```python
from build123d import *

# Parameters (mm, degrees)
SKETCH1_R           = 34.925
BOSS_EXTRUDE1_DEPTH = 3.175
CUT_EXTRUDE1_REACH  = 5.175
SKETCH2_R           = 2.413
CUT_EXTRUDE2_REACH  = 5.175
SKETCH4_R           = 1.9431
SKETCH4_R_2         = 0.762


with BuildPart() as part:
    # Sketch1 → Boss-Extrude1 (new body)
    with BuildSketch(Plane.XY):
        with Locations((67.638168, -28.60314574)):
            Circle(SKETCH1_R)
    extrude(amount=BOSS_EXTRUDE1_DEPTH)

    # Sketch2 → Cut-Extrude1 (cut, up to next)
    with BuildSketch(Plane.XY.offset(3.175), mode=Mode.PRIVATE) as cut_extrude1_sk1:
        with Locations((67.638168, 0)):
            Circle(SKETCH2_R)
    cut_extrude1_tool1 = extrude(cut_extrude1_sk1.sketch, amount=-CUT_EXTRUDE1_REACH, mode=Mode.PRIVATE) & part.part
    add(cut_extrude1_tool1.solids().sort_by_distance((67.638168, 0, 3.175))[0], mode=Mode.SUBTRACT)
    # Sketch2 → Cut-Extrude1 (cut, up to next)
    with BuildSketch(Plane.XY.offset(3.175), mode=Mode.PRIVATE) as cut_extrude1_sk2:
        with Locations((67.638168, -28.60314574)):
            Circle(SKETCH2_R)
    cut_extrude1_tool2 = extrude(cut_extrude1_sk2.sketch, amount=-CUT_EXTRUDE1_REACH, mode=Mode.PRIVATE) & part.part
    add(cut_extrude1_tool2.solids().sort_by_distance((67.638168, -28.603146, 3.175))[0], mode=Mode.SUBTRACT)

    # Sketch4 → Cut-Extrude2 (cut, up to next)
    with BuildSketch(Plane.XY.offset(3.175), mode=Mode.PRIVATE) as cut_extrude2_sk1:
        with Locations((54.938168, -28.60314574)):
            Circle(SKETCH4_R)
    cut_extrude2_tool1 = extrude(cut_extrude2_sk1.sketch, amount=-CUT_EXTRUDE2_REACH, mode=Mode.PRIVATE) & part.part
    add(cut_extrude2_tool1.solids().sort_by_distance((54.938168, -28.603146, 3.175))[0], mode=Mode.SUBTRACT)
    # Sketch4 → Cut-Extrude2 (cut, up to next)
    with BuildSketch(Plane.XY.offset(3.175), mode=Mode.PRIVATE) as cut_extrude2_sk2:
        with Locations((61.288168, -39.601668368)):
            Circle(SKETCH4_R_2)
    cut_extrude2_tool2 = extrude(cut_extrude2_sk2.sketch, amount=-CUT_EXTRUDE2_REACH, mode=Mode.PRIVATE) & part.part
    add(cut_extrude2_tool2.solids().sort_by_distance((61.288168, -39.601668, 3.175))[0], mode=Mode.SUBTRACT)
    # Sketch4 → Cut-Extrude2 (cut, up to next)
    with BuildSketch(Plane.XY.offset(3.175), mode=Mode.PRIVATE) as cut_extrude2_sk3:
        with Locations((80.338168, -28.60314574)):
            Circle(SKETCH4_R)
    cut_extrude2_tool3 = extrude(cut_extrude2_sk3.sketch, amount=-CUT_EXTRUDE2_REACH, mode=Mode.PRIVATE) & part.part
    add(cut_extrude2_tool3.solids().sort_by_distance((80.338168, -28.603146, 3.175))[0], mode=Mode.SUBTRACT)
    # Sketch4 → Cut-Extrude2 (cut, up to next)
    with BuildSketch(Plane.XY.offset(3.175), mode=Mode.PRIVATE) as cut_extrude2_sk4:
        with Locations((73.988168, -39.601668368)):
            Circle(SKETCH4_R_2)
    cut_extrude2_tool4 = extrude(cut_extrude2_sk4.sketch, amount=-CUT_EXTRUDE2_REACH, mode=Mode.PRIVATE) & part.part
    add(cut_extrude2_tool4.solids().sort_by_distance((73.988168, -39.601668, 3.175))[0], mode=Mode.SUBTRACT)


solid = part.part
```
Read the model definition and answer for the solid it produces. Units are mm, in the model's axes. Coordinates: 2 decimals unless noted, no trailing zeros. Loops run counter-clockwise (first coordinate to the right, second up) from the corner with the lowest first, then second, coordinate; pieces in that order, holes last.
(1) The mould has two halves that part along Y. Classify faces 1 (the face through (73.427, -39.087, 1.61)), 2 (the face through (61.7, -38.96, 1.61)), 3 (the face through (39.92, -49.85, 1.57)), 4 (the face through (67, -36, 0)): released by +Y, released by -Y, zero draft, split by the parting line, or undercut.
Solution:
face 1: undercut
face 2: undercut
face 3: split by the parting line
face 4: zero draft
(2) The part is cut by section C-C (x = 59.5). Determine the outline of the cut face in (y, z) (3 decimals).
Solution:
outline: (-62.567, 0) - (5.36, 0) - (5.36, 3.175) - (-62.567, 3.175) - close
(3) The part is cut by section B-B (z = 1.85). Determine the outline of the cut face in (x, y) (3 decimals).
Solution:
outline: circle Ø69.85 at (67.638, -28.603); hole circle Ø3.886 at (54.938, -28.603); hole circle Ø1.524 at (61.288, -39.602); hole circle Ø4.826 at (67.638, -28.603); hole circle Ø4.826 at (67.638, 0); hole circle Ø1.524 at (73.988, -39.602); hole circle Ø3.886 at (80.338, -28.603)
(4) Flat-ended cylindrical pins translate along their axes: pin 1 Ø2.5 at (x, y) = (80.34, -28.6) entering from +Z; pin 2 Ø1 at (y, z) = (-30, 0.5) entering from -X; pin 3 Ø1 at (x, z) = (84.5, 1) entering from -Y. Find the tip coordinate at first contact, or state that the pin passes through.
Solution:
pin 1: passes through
pin 2: stops at x = 32.72
pin 3: stops at y = -59.46
(5) Consider line 1 along Y through (x, z) = (80, 1.55); line 2 along X through (y, z) = (-52, 2.1); line 3 along X through (y, z) = (-37, 0.4). Determine where each line is inside the solid, lowest interval first.
Solution:
line 1: y = -61.27 to -30.52, -26.69 to 4.06
line 2: x = 41.71 to 93.57
line 3: x = 33.74 to 101.54
(6) The part is cut by section D-D (y = -8.5). Determine the outline of the cut face in (x, z) (3 decimals).
Solution:
outline: (39.079, 0) - (96.197, 0) - (96.197, 3.175) - (39.079, 3.175) - close
(7) The part is cut by section A-A (y = 0). Determine the outline of the cut face in (x, z) (3 decimals), and give its area (3 significant figures).
Solution:
outline: (47.598, 0) - (65.225, 0) - (65.225, 3.175) - (47.598, 3.175) - close; (70.051, 0) - (87.679, 0) - (87.679, 3.175) - (70.051, 3.175) - close
area: 112 mm2
